The model under review builds one solid part; all positions refer to its coordinate system, in mm. Face numbers are marked on the shaded views. A direction names the side the tool comes from. Give positions to 0.01 mm unless a question says otherwise; leave off trailing zeros. Order: outer loops, then holes, each group sorted by start corner. A loop starts at its lowest first (then second) coordinate and runs counter-clockwise, first axis right, second up. Notation, with made-up numbers: (83, -17) - (95, -17) arc R19 ccw to (95, -8) - close; hole circle Ø6 at (-21.75, 34). An arc over 180 degrees is marked (long way). Write item = value, one per line. Start each with the question number.
1. We need section A-A, the plane z = -6.5. State how many separate pieces and enclosed holes the cut face has, and give its area (3 significant figures).
2. Machinability: for the marked faces 1, 2, 3 and 4, which of the approach directions +Z, -Z, +X, -X, +Y, -Y give a long, thin tool a straight path to every point of the face, cutting with its end or side? Answer none if there is none.
3. We need section B-B, the plane y = 1.6. Give the boundary of the cut face in (x, z) (3 decimals).
4. Wall thickness on probe 1 along X at (y, z) = (14.75, 0); probe 2 along X at (y, z) = (25.75, 0); probe 3 along Z at (x, y) = (1.5, 26.75): over which ranges is each line inside the solid? List them lowest first.
5. For P1, Ø8, axis at x = 0, z = 0, coming from the +Y side; P2, Ø1.6, axis at x = 0, y = 1.6, coming from the +Z side; P3, Ø8, axis at y = 24.5, z = -5, coming from the +X side, all flat-tipped, find the tip position at first contact; note any pin that passes through.
6. Mouldability with a two-part tool opening along Y and no side actions: class the marked faces 5, 6 and 7 as pulls with the +Y half, pulls with the -Y half, needs draft (parallel to the pull), parting line crosses it, or undercut.
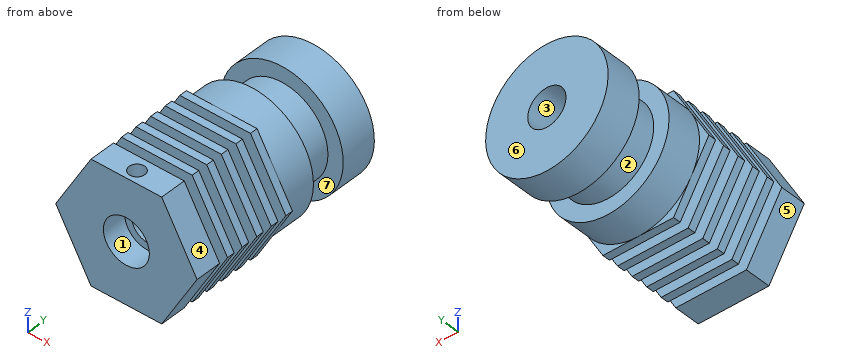
from build123d import *

# Parameters (mm, degrees)
SKETCH2_OUTSIDE_W            = 40.48
SKETCH2_OUTSIDE_H            = 40.48
CUT_EXTRUDE1_DEPTH           = 15.4
M6X1_0_TAPPED_HOLE1_D        = 5
M6X1_0_TAPPED_HOLE1_DEPTH    = 5
M6X1_0_TAPPED_HOLE1_TIP      = 1.502151548
M2_5X0_45_TAPPED_HOLE1_D     = 2.05
M2_5X0_45_TAPPED_HOLE1_DEPTH = 9
M2_5X0_45_TAPPED_HOLE1_TIP   = 0.615882135


with BuildPart() as part:
    # Sketch1 → Revolve1 (revolve)
    with BuildSketch(Plane.XY, mode=Mode.PRIVATE) as revolve1_sk:
        Polygon((3, 0), (3, 3.2), (2.05, 3.2), (2.05, 28.2), (8, 28.2), (8, 23.5), (6, 23.5), (6, 19), (8, 19), (8, 14.4), (14.307769621, 14.4), (14.307769621, 13.4), (4.75, 13.4), (4.75, 12.2), (14.307769621, 12.2), (14.307769621, 11.2), (4.75, 11.2), (4.75, 10), (14.307769621, 10), (14.307769621, 9), (4.75, 9), (4.75, 7.8), (14.307769621, 7.8), (14.307769621, 6.8), (4.75, 6.8), (4.75, 5.6), (14.307769621, 5.6), (14.307769621, 4.6), (4.75, 4.6), (4.75, 3.4), (14.307769621, 3.4), (14.307769621, 0), align=None)
    revolve(revolve1_sk.sketch.rotate(Axis((0, 0, 0), (0, 1, 0)), 90), axis=Axis((0, 0, 0), (0, 1, 0)))  # turned: the seam where the file's is

    # Sketch2 outside → Cut-Extrude1 (cut, through all)
    with BuildSketch(Plane(origin=(0, 14.4, 0), x_dir=(1, 0, 0), z_dir=(0, 1, 0))):
        Rectangle(SKETCH2_OUTSIDE_W, SKETCH2_OUTSIDE_H)
        Polygon((-4.618802154, 8), (-9.237604307, 0), (-4.618802154, -8), (4.618802154, -8), (9.237604307, 0), (4.618802154, 8), align=None, mode=Mode.SUBTRACT)
    extrude(amount=-CUT_EXTRUDE1_DEPTH, mode=Mode.SUBTRACT)

    # M6x1.0 Tapped Hole1
    with Locations(Plane(origin=(0, 28.2, 0), x_dir=(-1, 0, 0), z_dir=(0, 1, 0))):
        with Locations((0, 0)):
            Hole(M6X1_0_TAPPED_HOLE1_D / 2, depth=M6X1_0_TAPPED_HOLE1_DEPTH)
            with Locations((0, 0, -(M6X1_0_TAPPED_HOLE1_DEPTH + M6X1_0_TAPPED_HOLE1_TIP / 2))):  # 118° drill point
                Cone(0, M6X1_0_TAPPED_HOLE1_D / 2, M6X1_0_TAPPED_HOLE1_TIP, mode=Mode.SUBTRACT)

    # M2.5x0.45 Tapped Hole1
    with Locations(Plane.XY.offset(8)):
        with Locations((0, 1.6)):
            Hole(M2_5X0_45_TAPPED_HOLE1_D / 2, depth=M2_5X0_45_TAPPED_HOLE1_DEPTH)
            with Locations((0, 0, -(M2_5X0_45_TAPPED_HOLE1_DEPTH + M2_5X0_45_TAPPED_HOLE1_TIP / 2))):  # 118° drill point
                Cone(0, M2_5X0_45_TAPPED_HOLE1_D / 2, M2_5X0_45_TAPPED_HOLE1_TIP, mode=Mode.SUBTRACT)


solid = part.part
Model answer:
q1.separate_pieces = 7
q1.enclosed_holes = 0
q1.area = 179 mm2
q2.face_1 = -Y
q2.face_2 = none
q2.face_3 = +Y
q2.face_4 = +Z, +X, +Y, -Y
q3.outline = (-9.238, 0) - (-4.619, -8) - (4.619, -8) - (9.238, 0) - (4.619, 8) - (1.025, 8) - (1.025, 2.819) arc R3 cw (long way) to (-1.025, 2.819) - (-1.025, 8) - (-4.619, 8) - close
q4.probe_1 = -8 to -2.05, 2.05 to 8
q4.probe_2 = -8 to -2.5, 2.5 to 8
q4.probe_3 = -7.86 to -2, 2 to 7.86
q5.P1 = 28.2
q5.P2 = -2.89
q5.P3 = 7.94
q6.face_5 = needs draft
q6.face_6 = pulls with the +Y half
q6.face_7 = undercut
